```python
from build123d import *

# Parameters (mm, degrees)
SKETCH_1_R          = 60
EXTRUDE_1_DEPTH     = 120
SKETCH_3_R          = 7.5
EXTRUDE_3_DEPTH     = 350
SKETCH_4_R          = 10
CUT_EXTRUDE_1_DEPTH = 375.833296421
EXTRUDE_START       = 100
SKETCH_3_2_R        = 7.5
EXTRUDE_4_DEPTH     = 70


with BuildPart() as part:
    # 草图1 → 凸台-拉伸1 (new body)
    with BuildSketch(Plane.XY):
        Circle(SKETCH_1_R)
    extrude(amount=EXTRUDE_1_DEPTH)

    # 草图3 → 凸台-拉伸3 (add)
    with BuildSketch(Plane(origin=(0, 0, 0), x_dir=(0, 0, -1), z_dir=(1, 0, 0))):
        with Locations((-15, 0)):
            Circle(SKETCH_3_R)
    extrude(amount=-EXTRUDE_3_DEPTH)

    # 草图4 → 切除-拉伸1 (cut, through all)
    with BuildSketch(Plane.XY.offset(120)):
        Circle(SKETCH_4_R)
    extrude(amount=-CUT_EXTRUDE_1_DEPTH, mode=Mode.SUBTRACT)

    # 草图3<2> → 凸台-拉伸4 (add)
    with BuildSketch(Plane(origin=(0, 0, 0), x_dir=(0, 0, -1), z_dir=(1, 0, 0)).offset(EXTRUDE_START)):
        with Locations((-15, 0)):
            Circle(SKETCH_3_2_R)
    extrude(amount=-EXTRUDE_4_DEPTH)


solid = part.part
```
The listing builds one solid part. Answer for the finished solid, in the listing's coordinates (mm). A direction names the side the tool comes from. Give positions to 0.01 mm unless a question says otherwise; leave off trailing zeros. Order: outer loops, then holes, each group sorted by start corner. A loop starts at its lowest first (then second) coordinate and runs counter-clockwise, first axis right, second up. Notation, with made-up numbers: M 41,26 L 49,26 A14 ccw 49,37 Z; hole C -9,25.5 d3. An arc over 180 degrees is marked long. Put each result on its own line as item: value. Start each with the question number.
Item 1: For a pull along Y with two mould halves and no side action, classify faces 4 (the face through (55.425, -22.98, 59.16)), 5 (the face through (-2.17, -9.76, 60.84)), 6 (the face through (12, 1, 120)) as +Y half, -Y half, draft (parallel to the pull), parting line (faces both ways), or undercut.
Item 2: The part is cut by section A-A, the plane x = 0. Determine the outline of the cut face in (y, z).
Item 3: The part is cut by section C-C, the plane z = 15. Determine the outline of the cut face in (x, y), and give its area (3 significant figures).
Item 4: The part is cut by section B-B, the plane y = 0. Determine the outline of the cut face in (x, z), and give its area (4 significant figures).
Item 5: The part is cut by section D-D, the plane x = -119. Determine the outline of the cut face in (y, z).
Item 6: Flat-ended cylindrical pins translate along their axes: P1, Ø12, axis at y = -25, z = 32, coming from the -X side; P2, Ø8, axis at y = -22.5, z = 39, coming from the -X side; P3, Ø8, axis at y = 1.5, z = 64, coming from the -X side. Find the tip coordinate at first contact, or state that the pin passes through.
Item 7: Which of the six approach directions +Z, -Z, +X, -X, +Y, -Y give full straight-line access (tool end or side, diameter ignored) to faces 1 (the face through (80.048, 0.33, 22.493)), 2 (the face through (-350, 0, 15)), 3 (the face through (-202.731, 0.33, 22.493))?
Item 8: Find the intervals of material crossed by line 1 along Y through (x, z) = (0, 58); line 2 along Y through (x, z) = (-6.5, 25.5); line 3 along X through (y, z) = (-39, 95), in increasing order.
Answer key:
1. face 4: parting line
1. face 5: undercut
1. face 6: draft
2. outline: M -60,0 L -10,0 L -10,120 L -60,120 Z; M 10,0 L 60,0 L 60,120 L 10,120 Z
3. outline: M -350,-7.5 L -59.53,-7.5 A60 ccw 59.53,-7.5 L 100,-7.5 L 100,7.5 L 59.53,7.5 A60 ccw -59.53,7.5 L -350,7.5 Z; hole C 0,0 d20
3. area: 16,000 mm²
4. outline: M -350,7.5 L -60,7.5 L -60,0 L -10,0 L -10,120 L -60,120 L -60,22.5 L -350,22.5 Z; M 10,0 L 60,0 L 60,7.5 L 100,7.5 L 100,22.5 L 60,22.5 L 60,120 L 10,120 Z
4. area: 16,950 mm²
5. outline: C 0,15 d15
6. P1: stops at x = -56.91
6. P2: stops at x = -57.08
6. P3: stops at x = -60
7. face 1: +X
7. face 2: +Z, -Z, -X, +Y, -Y
7. face 3: -X
8. line 1: y = -60 to -10, 10 to 60
8. line 2: y = -59.65 to -7.6, 7.6 to 59.65
8. line 3: x = -45.6 to 45.6
